Build history of the part. All positions in model axes, mm. A direction names the side the tool comes from. Coordinates: 2 decimals unless noted, no trailing zeros. Write each loop counter-clockwise with the first axis right and the second up, starting at its lowest first coordinate (ties: lowest second). Pieces come first, ordered by that corner, then holes. Notation, with made-up numbers: (47.25, 7) -> (76.25, 7) arc R23 ccw to (76.25, 40) -> close; hole circle Ø11 at (88.25, -9). An arc over 180 degrees is marked (long way). Write each question's results on one line, items separated by ' | '. Start each with the question number.
Q1. Saw through at C-C on z = -27.5. Give the cut face in (x, y).
Q2. Drill centre lines: line 1 (X direction, y = 12.5, z = -0.5); line 2 (Z direction, x = 0, y = 24); line 3 (X direction, y = 2, z = 3.5). Where is each one in solid material? Low to high.
Q3. Saw through at B-B on z = 7.5. Give the cut face in (x, y).
Q4. Drop flat-ended pins along their axis: pin 1 Ø2.5 at (x, y) = (-23, 3.5) entering from -Z; pin 2 Ø4 at (x, y) = (23, 3) entering from -Z; pin 3 Ø1.5 at (y, z) = (23.5, 7.5) entering from +X; pin 4 Ø24 at (x, z) = (0, 0) entering from -Y. Give the stop position or say it passes through.
Q5. Two-plate mould, pull along X, no slides. Class faces 1 (the face through (5, 0, -10)), 2 (the face through (-22, 4, -2)), 3 (the face through (7.19, 3.94, 32.36)), 4 (the face through (-22, 4, 2)): released by +X, released by -X, zero draft, split by the parting line, or undercut.
Q6. Tool access for faces 5 (the face through (-6.691, 16.269, 12.864)), 6 (the face through (-20.415, 3.944, 20.829)), 7 (the face through (-10, 33, 4)): list every direction of +Z, -Z, +X, -X, +Y, -Y with a clear straight run to the whole face (end or side of a thin tool).
Q7. Saw through at D-D on x = -7.5. Give the cut face in (y, z), and give its area (3 significant figures).
Q8. Saw through at A-A on x = 0. Give the cut face in (y, z).
Autodesk Inventor part; units mm, degrees
ref_plane "YZ Plane" through (0, 0, 0) normal (1, 0, 0) x (0, 1, 0)
ref_plane "XZ Plane" through (0, 0, 0) normal (0, 1, 0) x (-1, 0, 0)
ref_plane "XY Plane" through (0, 0, 0) normal (0, 0, 1) x (1, 0, 0)
sketch "Sketch1" plane through (0, 0, 0) normal (0, 1, 0) x (-1, 0, 0)
  circle A0 centre (0, 0) radius 33.15
  circle A1 centre (0, 0) radius 29.165
  circle A2 centre (0, 0) radius 10.5
  circle A3 centre (0, 0) radius 14.5
  dimension "d0" = 66.3
  dimension "d1" = 58.33
  dimension "d2" = 21
  dimension "d3" = 29
sketch "Sketch2" plane through (0, 0, 0) normal (0, 1, 0) x (-1, 0, 0)
  line L0 (2, 33) -> (-2, 33)
  line L1 (-2, 33) -> (-2, 12)
  line L2 (-2, 12) -> (2, 12)
  line L3 (2, 12) -> (2, 33)
  line L4 (33, 2) -> (12, 2)
  line L5 (12, 2) -> (12, -2)
  line L6 (12, -2) -> (33, -2)
  line L7 (33, -2) -> (33, 2)
  line L8 (2, -12) -> (-2, -12)
  line L9 (-2, -12) -> (-2, -33)
  line L10 (-2, -33) -> (2, -33)
  line L11 (2, -33) -> (2, -12)
  line L12 (-12, 2) -> (-33, 2)
  line L13 (-33, 2) -> (-33, -2)
  line L14 (-33, -2) -> (-12, -2)
  line L15 (-12, -2) -> (-12, 2)
  point P0 (0, 0)
  point P1 (12, 0)
  point P2 (0, -12)
  point P3 (-33, 0)
  dimension "d4" = 4
  dimension "d5" = 4
  dimension "d6" = 12
  dimension "d7" = 12
  dimension "d8" = 12
  dimension "d9" = 12
  dimension "d10" = 21
  dimension "d11" = 21
  dimension "d12" = 21
  dimension "d13" = 21
  dimension "d14" = 2
  dimension "d15" = 2
extrude "Extrusion1" add sketch "Sketch1" along normal blind 8
extrude "Extrusion2" add sketch "Sketch2" along normal blind 8
extrude "Extrusion3" add sketch "Sketch1" along normal blind 33 contours A3
equation "\"d11\" = d10"
equation "\"d12\" = d10"
properties part number "Calibrator"
Returned:
1) outline: (-18.51, 0) -> (-9.71, 0) -> (-9.71, 8) -> (-18.51, 8) -> close; (-2, 0) -> (2, 0) -> (2, 8) -> (-2, 8) -> close; (9.71, 0) -> (18.51, 0) -> (18.51, 8) -> (9.71, 8) -> close
2) line 1: x = -14.49 to -10.49, 10.49 to 14.49 | line 2: z = -14.5 to -10.5, 10.5 to 14.5 | line 3: x = -32.96 to -28.95, -14.07 to -9.9, 9.9 to 14.07, 28.95 to 32.96
3) outline: (-32.29, 0) -> (-28.18, 0) -> (-28.18, 8) -> (-32.29, 8) -> close; (-12.41, 0) -> (-7.35, 0) -> (-7.35, 33) -> (-12.41, 33) -> close; (7.35, 0) -> (12.41, 0) -> (12.41, 33) -> (7.35, 33) -> close; (28.18, 0) -> (32.29, 0) -> (32.29, 8) -> (28.18, 8) -> close
4) pin 1: stops at z = -25.02 | pin 2: stops at z = -25.65 | pin 3: stops at x = 12.83 | pin 4: stops at y = 0
5) face 1: zero draft | face 2: undercut | face 3: split by the parting line | face 4: undercut
6) face 5: +Y | face 6: +Y, -Y | face 7: +Z, -Z, +X, -X, +Y
7) outline: (0, -32.29) -> (8, -32.29) -> (8, -28.18) -> (0, -28.18) -> close; (0, -12.41) -> (33, -12.41) -> (33, -7.35) -> (0, -7.35) -> close; (0, 7.35) -> (33, 7.35) -> (33, 12.41) -> (0, 12.41) -> close; (0, 28.18) -> (8, 28.18) -> (8, 32.29) -> (0, 32.29) -> close | area: 400 mm2
8) outline: (0, -33.15) -> (8, -33.15) -> (8, -14.5) -> (33, -14.5) -> (33, -10.5) -> (0, -10.5) -> close; (0, 10.5) -> (33, 10.5) -> (33, 14.5) -> (8, 14.5) -> (8, 33.15) -> (0, 33.15) -> close
